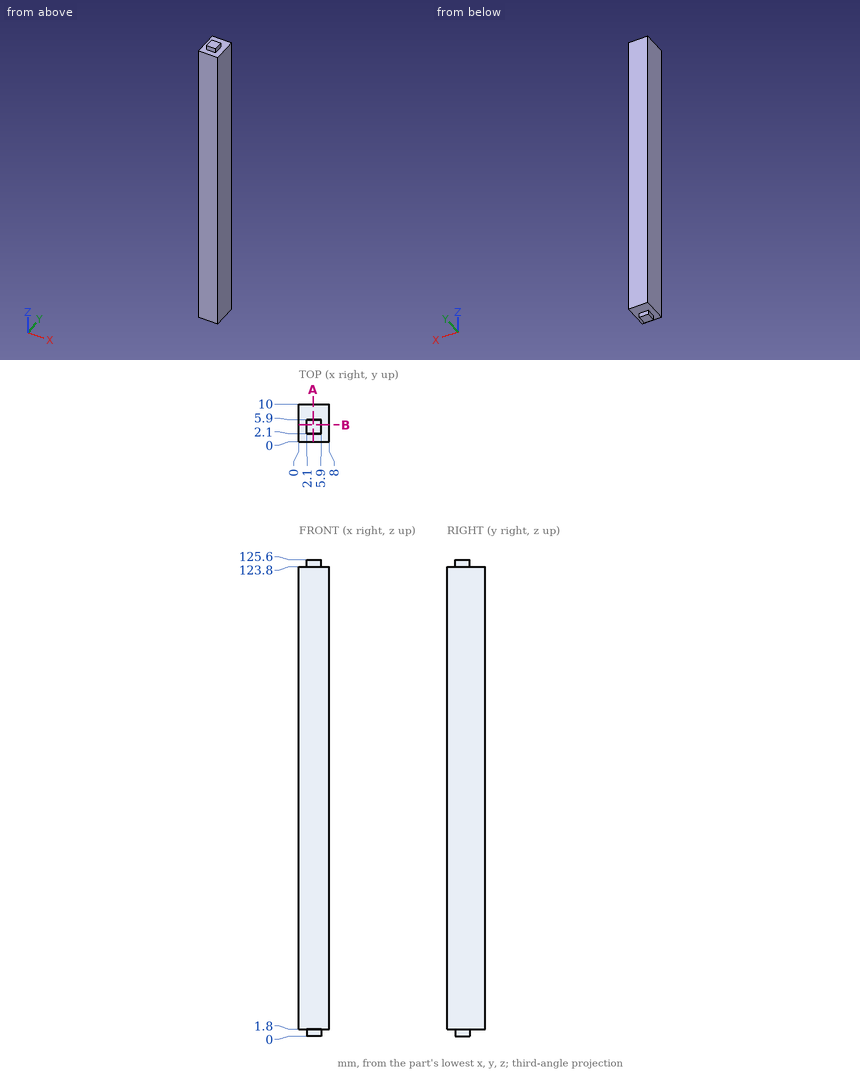
Verification items for this drawing (mm, ordinates from the low corner). Round coordinates to 2 decimals unless told otherwise and drop trailing zeros. Write each loop counter-clockwise with the first axis right and the second up, starting at its lowest first coordinate (ties: lowest second). Pieces come first, ordered by that corner, then holes. Notation, with made-up numbers: (68.25, 81) - (84.25, 81) arc R11 ccw to (84.25, 101) - close; hole circle Ø6 at (76, -4). An arc over 180 degrees is marked (long way). One line per item, written item: value.
1. Scan line: L1, parallel to Z at x = 4.25, y = 9.25. Record every from-to range of solid material in increasing order.
The answers:
L1: z = 1.8 to 123.8
2. Depth check by flat-ended pin: pin 1 Ø0.9 at (y, z) = (4.5, 124.5) entering from +X; pin 2 Ø1.4 at (x, z) = (5, 125) entering from +Y; pin 3 Ø0.5 at (y, z) = (5, 124.5) entering from -X; pin 4 Ø2 at (x, z) = (4.5, 124.5) entering from -Y. Enter the tip coordinate at first touch or a pass-through.
The answers:
pin 1: stops at x = 5.9
pin 2: stops at y = 5.9
pin 3: stops at x = 2.1
pin 4: stops at y = 0
3. Cross-section at B-B on y = 4.5. Record the boundary of the cut face in (x, z), and give its area (3 significant figures).
The answers:
outline: (0, 1.8) - (2.1, 1.8) - (2.1, 0) - (5.9, 0) - (5.9, 1.8) - (8, 1.8) - (8, 123.8) - (5.9, 123.8) - (5.9, 125.6) - (2.1, 125.6) - (2.1, 123.8) - (0, 123.8) - close
area: 990 mm^2
4. Cross-section at A-A on x = 3.75. Record the boundary of the cut face in (y, z).
The answers:
outline: (0, 1.8) - (2.1, 1.8) - (2.1, 0) - (5.9, 0) - (5.9, 1.8) - (10, 1.8) - (10, 123.8) - (5.9, 123.8) - (5.9, 125.6) - (2.1, 125.6) - (2.1, 123.8) - (0, 123.8) - close
